from build123d import *

# Parameters (mm, degrees)
F2_DEPTH  = 82
F3_DEPTH  = 10
F4_START  = -72
F4_DEPTH  = 10
F7_DEPTH  = 10
F8_START  = 102.8
F8_DEPTH  = 10
F10_R     = 13.5
F11_DEPTH = 1.6
F12_W     = 13
F12_H     = 12
F13_DEPTH = 1.6


# Not quite as in the source:
# - a feature names something its author has since deleted; it is built from what else it names


with BuildPart() as f2:
    # F1 (on offset) → F2 (new body)
    with BuildSketch(Plane.XZ.offset(41)):
        Polygon((78.5, 0), (78.5, 1.6), (-78.5, 1.6), (-78.5, 0), (-73.5, 0), (-71.9, 0), (-66.9, 0), (-39.1, 0), (-34.1, 0), (-32.5, 0), (-27.5, 0), (27.5, 0), (32.5, 0), (34.1, 0), (39.1, 0), (66.9, 0), (71.9, 0), (73.5, 0), align=None)
    extrude(amount=-F2_DEPTH)

    # F1 (on offset) → F3 (join)
    with BuildSketch(Plane.XZ.offset(41)):
        Polygon((-66.9, 0), (-71.9, 0), (-71.9, -5), align=None)
        Polygon((-34.1, 0), (-39.1, 0), (-34.1, -5), align=None)
        Polygon((-27.5, 0), (-32.5, 0), (-32.5, -5), align=None)
        Polygon((-73.5, 0), (-78.5, 0), (-73.5, -5), align=None)
    extrude(amount=-F3_DEPTH)

    # F1 (on offset) → F4 (join)
    with BuildSketch(Plane.XZ.offset(41).offset(F4_START)):
        Polygon((-66.9, 0), (-71.9, 0), (-71.9, -5), align=None)
        Polygon((-34.1, 0), (-39.1, 0), (-34.1, -5), align=None)
        Polygon((-27.5, 0), (-32.5, 0), (-32.5, -5), align=None)
        Polygon((-73.5, 0), (-78.5, 0), (-73.5, -5), align=None)
    extrude(amount=-F4_DEPTH)

    # F6 (on offset) → F7 (join)
    with BuildSketch(Plane.YZ.offset(-51.4)):
        Polygon((-11.1, 0), (-11.1, -5), (-6.1, 0), align=None)
        Polygon((-14.3, -5), (-14.3, 0), (-19.3, 0), align=None)
    extrude(amount=-F7_DEPTH)

    # F6 (on offset) → F8 (join)
    with BuildSketch(Plane.YZ.offset(-51.4).offset(F8_START)):
        Polygon((-11.1, 0), (-11.1, -5), (-6.1, 0), align=None)
        Polygon((-14.3, -5), (-14.3, 0), (-19.3, 0), align=None)
    extrude(amount=F8_DEPTH)

    # F9: F2 across plane


with BuildPart() as f2_1:
    add(f2.part)
    add(f2.part.mirror(Plane.YZ))

    # F10 (on face) → F11 (cut)
    with BuildSketch(Plane.XY.offset(1.6)):
        with Locations((0, -17.0082943066)):
            Circle(F10_R)
    extrude(amount=-F11_DEPTH, mode=Mode.SUBTRACT)

    # F12 (on face) → F13 (cut)
    with BuildSketch(Plane.XY.offset(1.6)):
        with Locations((-26.0217403993, 18.549364836)):
            Rectangle(F12_W, F12_H)
        with Locations((26.0217403993, 18.549364836)):
            Rectangle(F12_W, F12_H)
    extrude(amount=-F13_DEPTH, mode=Mode.SUBTRACT)


solid = f2_1.part
Read the model definition and answer for the solid it produces. Units are mm, in the model's axes. A direction names the side the tool comes from. Round coordinates to 2 decimals unless told otherwise and drop trailing zeros. Loops run counter-clockwise (first coordinate to the right, second up) from the corner with the lowest first, then second, coordinate; pieces in that order, holes last.
Q1. Each of these flat-tipped pins is pushed along its axis until it touches: pin 1 (1.5 mm diameter, centred on x = -55, z = -3.5, fed in from -Y); pin 2 (1.5 mm diameter, centred on y = -8.5, z = -3, fed in from -X); pin 3 (2.5 mm diameter, centred on y = -18, z = -1.5, fed in from +X). Where does it stop, or does it pass through?
Q2. Consider probe 1 along Y at (x, z) = (0, 1.1); probe 2 along Z at (x, y) = (57, -26); probe 3 along X at (y, z) = (-24.5, 0.5). Determine where each line is inside the solid, lowest interval first.
Q3. Section B-B on x = 0 is taken. Write down the section's boundary in (y, z), and give its area (3 significant figures).
Q4. Section C-C on y = -33.5 is taken. Write down the section's boundary in (x, z), and give its area (3 significant figures).
Q5. Section A-A on y = 14.5 is taken. Write down the section's boundary in (x, z), and give its area (3 significant figures).
Q6. Section D-D on z = -3.25 is taken. Give the number of separate pieces and of enclosed holes in the cut face, and give its area (3 significant figures).
Q7. Determine the mould class of faces 1 (the face through (-61.4, -16, -1)), 2 (the face through (-75, -31, -1)), 3 (the face through (-73.5, 36, -3)) for opening direction X: released by +X, released by -X, zero draft, split by the parting line, or undercut.
Q8. Which of the six approach directions +Z, -Z, +X, -X, +Y, -Y give full straight-line access (tool end or side, diameter ignored) to faces 4 (the face through (-71.9, 36, -2)), 5 (the face through (-31, 31, -2)), 6 (the face through (-61.4, -9, -2))?
Output:
1. pin 1: stops at y = -16.55
1. pin 2: stops at x = -61.4
1. pin 3: stops at x = 61.4
2. probe 1: y = -41 to -30.51, -3.51 to 41
2. probe 2: z = 0 to 1.6
2. probe 3: x = -78.5 to -11.23, 11.23 to 78.5
3. outline: (-41, 0) - (-30.51, 0) - (-30.51, 1.6) - (-41, 1.6) - close; (-3.51, 0) - (41, 0) - (41, 1.6) - (-3.51, 1.6) - close
3. area: 88.0 mm2
4. outline: (-78.5, 0) - (-73.5, -5) - (-73.5, 0) - (-71.9, 0) - (-71.9, -5) - (-66.9, 0) - (-39.1, 0) - (-34.1, -5) - (-34.1, 0) - (-32.5, 0) - (-32.5, -5) - (-27.5, 0) - (27.5, 0) - (32.5, -5) - (32.5, 0) - (34.1, 0) - (34.1, -5) - (39.1, 0) - (66.9, 0) - (71.9, -5) - (71.9, 0) - (73.5, 0) - (73.5, -5) - (78.5, 0) - (78.5, 1.6) - (-78.5, 1.6) - close
4. area: 351 mm2
5. outline: (-78.5, 0) - (-32.52, 0) - (-32.52, 1.6) - (-78.5, 1.6) - close; (-19.52, 0) - (19.52, 0) - (19.52, 1.6) - (-19.52, 1.6) - close; (32.52, 0) - (78.5, 0) - (78.5, 1.6) - (32.52, 1.6) - close
5. area: 210 mm2
6. separate pieces: 20
6. enclosed holes: 0
6. area: 350 mm2
7. face 1: released by -X
7. face 2: zero draft
7. face 3: undercut
8. face 4: -Z, +Y, -Y
8. face 5: -Z, +X, -X
8. face 6: -Z, -X, +Y, -Y
